Source: CAD feature listing. Evaluate the final solid. Frame: model axes, mm. Give positions to 0.01 mm unless a question says otherwise; leave off trailing zeros. Order: outer loops, then holes, each group sorted by start corner. A loop starts at its lowest first (then second) coordinate and runs counter-clockwise, first axis right, second up. Notation, with made-up numbers: M -10,59.5 L 44,59.5 A22 ccw 44,84.5 Z; hole C -25.5,47.5 d2. An arc over 180 degrees is marked long. Answer as a JSON object with one key per item and string values. Group by question number.
1. Section query A-A (x = -12.5). Output: boundary loops of the cut face in (y, z), plus the area to 3 significant figures.
2. Material intervals for L1, parallel to X at y = -1, z = 20; L2, parallel to Y at x = 22.5, z = -33, sorted ascending. Write a range as [from, to].
3. Section query B-B (y = -2.75). Output: boundary loops of the cut face in (x, z).
4. Section query C-C (z = 6). Output: boundary loops of the cut face in (x, y), plus the area to 3 significant figures.
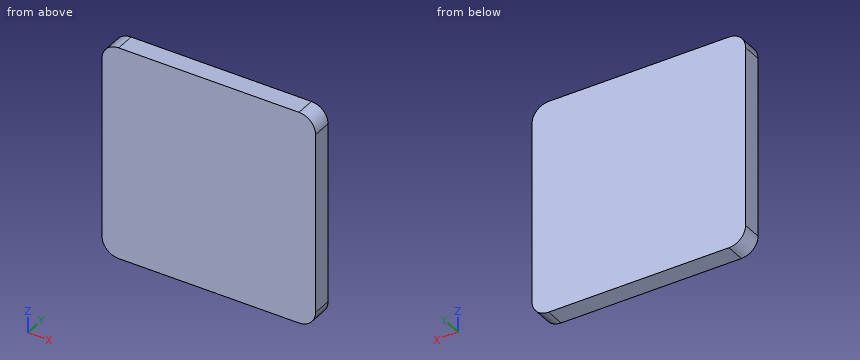
from build123d import *

# Parameters (mm, degrees)
F1_DEPTH = 5
F3_DEPTH = 1
F5_DEPTH = 1


with BuildPart() as f1:
    # F0 (on Front) → F1 (new body)
    with BuildSketch(Plane.XZ):
        with BuildLine():
            Line((-32.5, -38.5), (32.5, -38.5))
            ThreePointArc((32.5, -38.5), (36.7426406871, -36.7426406871), (38.5, -32.5))
            Line((38.5, -32.5), (38.5, 32.5))
            ThreePointArc((38.5, 32.5), (36.7426406871, 36.7426406871), (32.5, 38.5))
            Line((32.5, 38.5), (-32.5, 38.5))
            ThreePointArc((-32.5, 38.5), (-36.7426406871, 36.7426406871), (-38.5, 32.5))
            Line((-38.5, 32.5), (-38.5, -32.5))
            ThreePointArc((-38.5, -32.5), (-36.7426406871, -36.7426406871), (-32.5, -38.5))
        make_face()
        with BuildLine():
            ThreePointArc((37.5, -32.5), (36.0355339059, -36.0355339059), (32.5, -37.5))
            Line((32.5, -37.5), (-32.5, -37.5))
            ThreePointArc((-32.5, -37.5), (-36.0355339059, -36.0355339059), (-37.5, -32.5))
            Line((-37.5, -32.5), (-37.5, 32.5))
            ThreePointArc((-37.5, 32.5), (-36.0355339059, 36.0355339059), (-32.5, 37.5))
            Line((-32.5, 37.5), (32.5, 37.5))
            ThreePointArc((32.5, 37.5), (36.0355339059, 36.0355339059), (37.5, 32.5))
            Line((37.5, 32.5), (37.5, -32.5))
        make_face(mode=Mode.SUBTRACT)
    extrude(amount=F1_DEPTH)

    # F2 (on face) → F3 (join)
    with BuildSketch(Plane.XZ.offset(5)):
        with BuildLine():
            ThreePointArc((-38.5, -32.5), (-36.7426406871, -36.7426406871), (-32.5, -38.5))
            Line((-32.5, -38.5), (32.5, -38.5))
            ThreePointArc((32.5, -38.5), (36.7426406871, -36.7426406871), (38.5, -32.5))
            Line((38.5, -32.5), (38.5, 32.5))
            ThreePointArc((38.5, 32.5), (36.7426406871, 36.7426406871), (32.5, 38.5))
            Line((32.5, 38.5), (-32.5, 38.5))
            ThreePointArc((-32.5, 38.5), (-36.7426406871, 36.7426406871), (-38.5, 32.5))
            Line((-38.5, 32.5), (-38.5, -32.5))
        make_face()
        with BuildLine():
            Line((37.5, 32.5), (37.5, -32.5))
            ThreePointArc((37.5, -32.5), (36.0355339059, -36.0355339059), (32.5, -37.5))
            Line((32.5, -37.5), (-32.5, -37.5))
            ThreePointArc((-32.5, -37.5), (-36.0355339059, -36.0355339059), (-37.5, -32.5))
            Line((-37.5, -32.5), (-37.5, 32.5))
            ThreePointArc((-37.5, 32.5), (-36.0355339059, 36.0355339059), (-32.5, 37.5))
            Line((-32.5, 37.5), (32.5, 37.5))
            ThreePointArc((32.5, 37.5), (36.0355339059, 36.0355339059), (37.5, 32.5))
        make_face(mode=Mode.SUBTRACT)
        with BuildLine():
            ThreePointArc((32.5, -37.5), (36.0355339059, -36.0355339059), (37.5, -32.5))
            Line((37.5, -32.5), (37.5, 32.5))
            ThreePointArc((37.5, 32.5), (36.0355339059, 36.0355339059), (32.5, 37.5))
            Line((32.5, 37.5), (-32.5, 37.5))
            ThreePointArc((-32.5, 37.5), (-36.0355339059, 36.0355339059), (-37.5, 32.5))
            Line((-37.5, 32.5), (-37.5, -32.5))
            ThreePointArc((-37.5, -32.5), (-36.0355339059, -36.0355339059), (-32.5, -37.5))
            Line((-32.5, -37.5), (32.5, -37.5))
        make_face()
    extrude(amount=F3_DEPTH)

    # F4 (on face) → F5 (join)
    with BuildSketch(Plane(origin=(0, 0, 0), x_dir=(-1, 0, 0), z_dir=(0, 1, 0))):
        with BuildLine():
            ThreePointArc((-38.5, -32.5), (-36.7426406871, -36.7426406871), (-32.5, -38.5))
            Line((-32.5, -38.5), (32.5, -38.5))
            ThreePointArc((32.5, -38.5), (36.7426406871, -36.7426406871), (38.5, -32.5))
            Line((38.5, -32.5), (38.5, 32.5))
            ThreePointArc((38.5, 32.5), (36.7426406871, 36.7426406871), (32.5, 38.5))
            Line((32.5, 38.5), (-32.5, 38.5))
            ThreePointArc((-32.5, 38.5), (-36.7426406871, 36.7426406871), (-38.5, 32.5))
            Line((-38.5, 32.5), (-38.5, -32.5))
        make_face()
        with BuildLine():
            Line((32.5, -37.5), (-32.5, -37.5))
            ThreePointArc((-32.5, -37.5), (-36.0355339059, -36.0355339059), (-37.5, -32.5))
            Line((-37.5, -32.5), (-37.5, 32.5))
            ThreePointArc((-37.5, 32.5), (-36.0355339059, 36.0355339059), (-32.5, 37.5))
            Line((-32.5, 37.5), (32.5, 37.5))
            ThreePointArc((32.5, 37.5), (36.0355339059, 36.0355339059), (37.5, 32.5))
            Line((37.5, 32.5), (37.5, -32.5))
            ThreePointArc((37.5, -32.5), (36.0355339059, -36.0355339059), (32.5, -37.5))
        make_face(mode=Mode.SUBTRACT)
        with BuildLine():
            ThreePointArc((-37.5, -32.5), (-36.0355339059, -36.0355339059), (-32.5, -37.5))
            Line((-32.5, -37.5), (32.5, -37.5))
            ThreePointArc((32.5, -37.5), (36.0355339059, -36.0355339059), (37.5, -32.5))
            Line((37.5, -32.5), (37.5, 32.5))
            ThreePointArc((37.5, 32.5), (36.0355339059, 36.0355339059), (32.5, 37.5))
            Line((32.5, 37.5), (-32.5, 37.5))
            ThreePointArc((-32.5, 37.5), (-36.0355339059, 36.0355339059), (-37.5, 32.5))
            Line((-37.5, 32.5), (-37.5, -32.5))
        make_face()
    extrude(amount=F5_DEPTH)


solid = f1.part
Answer sheet:
{
 "1": {"outline": "M -6,-38.5 L 1,-38.5 L 1,38.5 L -6,38.5 Z; hole M -5,-37.5 L 0,-37.5 L 0,37.5 L -5,37.5 Z", "area": "164 mm^2"},
 "2": {"L1": "[-38.5, -37.5], [37.5, 38.5]", "L2": "[-6, -5], [0, 1]"},
 "3": {"outline": "M -38.5,-32.5 A6 ccw -32.5,-38.5 L 32.5,-38.5 A6 ccw 38.5,-32.5 L 38.5,32.5 A6 ccw 32.5,38.5 L -32.5,38.5 A6 ccw -38.5,32.5 Z; hole M -37.5,-32.5 A5 ccw -32.5,-37.5 L 32.5,-37.5 A5 ccw 37.5,-32.5 L 37.5,32.5 A5 ccw 32.5,37.5 L -32.5,37.5 A5 ccw -37.5,32.5 Z"},
 "4": {"outline": "M -38.5,-6 L 38.5,-6 L 38.5,1 L -38.5,1 Z; hole M -37.5,-5 L 37.5,-5 L 37.5,0 L -37.5,0 Z", "area": "164 mm^2"}
}
